```python
from build123d import *

# Parameters (mm, degrees)
SKETCH1_R           = 13.4
BOSS_EXTRUDE1_DEPTH = 56
SKETCH2_W           = 100
SKETCH2_H           = 60
BOSS_EXTRUDE2_DEPTH = 4
SKETCH3_R           = 13.4
CUT_EXTRUDE1_DEPTH  = 25.2
SKETCH4_W           = 25.2
SKETCH4_H           = 25.2
CUT_EXTRUDE2_DEPTH  = 51.2
FILLET1_R           = 5
FILLET2_R           = 5
FILLET4_R           = 3
FILLET5_R           = 3


with BuildPart() as part:
    # Sketch1 → Boss-Extrude1 (new body)
    with BuildSketch(Plane(origin=(0, 0, 0), x_dir=(1, 0, 0), z_dir=(0, 1, 0))):
        Polygon((-65.2, -11.320132013), (-65.2, 44.679867987), (0, 44.679867987), (0, 48.679867987), (-100, 48.679867987), (-100, -11.320132013), align=None)
        with Locations(Location((-82.6, 31.279867987, 0), (0, 0, 270))):
            Circle(SKETCH1_R, mode=Mode.SUBTRACT)
    boss_extrude1 = extrude(amount=BOSS_EXTRUDE1_DEPTH)

    # Sketch2 → Boss-Extrude2 (add)
    with BuildSketch(Plane(origin=(0, 0, 0), x_dir=(1, 0, 0), z_dir=(0, 1, 0))):
        with Locations((-50, 18.679867987)):
            Rectangle(SKETCH2_W, SKETCH2_H)
    boss_extrude2 = extrude(amount=-BOSS_EXTRUDE2_DEPTH)

    # Sketch3 → Cut-Extrude1 (cut)
    with BuildSketch(Plane.XY.offset(11.320132013)):
        with Locations((-82.6, 13.4)):
            Circle(SKETCH3_R)
    cut_extrude1 = extrude(amount=-CUT_EXTRUDE1_DEPTH, mode=Mode.SUBTRACT)

    # Sketch4 → Cut-Extrude2 (cut)
    with BuildSketch(Plane.ZY.offset(100)):
        with Locations((-1.279867987, 43.4)):
            Rectangle(SKETCH4_W, SKETCH4_H)
    cut_extrude2 = extrude(amount=-CUT_EXTRUDE2_DEPTH, mode=Mode.SUBTRACT)

    # Mirror2: Boss-Extrude1, Boss-Extrude2, Cut-Extrude1, Cut-Extrude2 across plane
    add(boss_extrude1.mirror(Plane.ZY))
    add(boss_extrude2.mirror(Plane.ZY))
    add(cut_extrude1.mirror(Plane.ZY), mode=Mode.SUBTRACT)
    add(cut_extrude2.mirror(Plane.ZY), mode=Mode.SUBTRACT)

    # Fillet1
    fillet1_edges = [part.edges().sort_by_distance(p)[0] for p in [
        (0, 0, -44.679867987),
        (-65.2, 0, -16.679867987),
        (-65.2, 28, -44.679867987),
        (65.2, 0, -16.679867987),
        (65.2, 28, -44.679867987),
    ]]
    fillet(fillet1_edges, radius=FILLET1_R)

    # Fillet2
    fillet2_edges = [part.edges().sort_by_distance(p)[0] for p in [
        (-100, 26, -48.679867987),
        (-100, -4, -18.679867987),
        (0, -4, -48.679867987),
        (100, 26, -48.679867987),
        (100, -4, -18.679867987),
    ]]
    fillet(fillet2_edges, radius=FILLET2_R)

    # Fillet4
    fillet4_edges = [part.edges().sort_by_distance(p)[0] for p in [
        (-65.2, 30.8, -1.279867987),
        (-65.2, 43.4, -13.879867987),
        (-82.6, 30.8, -13.879867987),
        (-100, 43.4, -13.879867987),
        (-100, 30.8, -1.279867987),
    ]]
    fillet(fillet4_edges, radius=FILLET4_R)

    # Fillet5
    fillet5_edges = [part.edges().sort_by_distance(p)[0] for p in [
        (100, 43.4, -13.879867987),
        (82.6, 30.8, -13.879867987),
        (100, 30.8, -1.279867987),
        (65.2, 43.4, -13.879867987),
        (65.2, 30.8, -1.279867987),
    ]]
    fillet(fillet5_edges, radius=FILLET5_R)


solid = part.part
```
The model under review builds one solid part; all positions refer to its coordinate system, in mm. A direction names the side the tool comes from. Round coordinates to 2 decimals unless told otherwise and drop trailing zeros. Loops run counter-clockwise (first coordinate to the right, second up) from the corner with the lowest first, then second, coordinate; pieces in that order, holes last. Notation, with made-up numbers: (35.5, 79.5) -> (63.5, 79.5) arc R25 cw to (63.5, 118.5) -> close; hole circle Ø5 at (27.25, 88.5). An arc over 180 degrees is marked (long way). Answer as a JSON object with one key per item and string values. Group by question number.
1) We need section C-C on x = -40. Write out the cut boundary in (y, z).
2) For line 1 (X direction, y = 13, z = -8); line 2 (Z direction, x = 82, y = 42); line 3 (X direction, y = 14, z = -26), list the stretches that pass through material, from the lowest coordinate up. Write a range as [from, to].
3) For pin 1 Ø21.5 at (x, y) = (-82.5, 16) entering from +Z; pin 2 Ø5 at (x, z) = (-75.5, -23.5) entering from +Y; pin 3 Ø8 at (y, z) = (29, -13) entering from -X; pin 4 Ø15.5 at (x, y) = (-29.5, 29) entering from +Z, all flat-tipped, find the tip position at first contact; note any pin that passes through.
4) We need section B-B on z = -8.5. Write out the cut boundary in (x, y), then the cut area to 3 significant figures.
5) For faces 4 (the face through (83, 30.8, 0)), 5 (the face through (1, 0, -15)), 6 (the face through (83, 0, -31)), list the 3-axis set-ups (+Z, -Z, +X, -X, +Y, -Y) from which the entire face can be reached by the end or side of a thin tool; tool diameter is ignored.
6) We need section A-A on y = 49. Write out the cut boundary in (x, z).
7) Mouldability with a two-part tool opening along Z and no side actions: class faces 1 (the face through (1, 29, -48.68)), 2 (the face through (-73.544, 27.608, -41.156)), 3 (the face through (-69.819, 17.425, -1.103)) as released by +Z, released by -Z, zero draft, split by the parting line, or undercut.
8) We need section D-D on z = -26. Write out the cut boundary in (x, y), then the cut area to 3 significant figures.
Result set:
{
 "1": {"outline": "(-4, -43.68) arc R5 ccw to (1, -48.68) -> (56, -48.68) -> (56, -44.68) -> (5, -44.68) arc R5 cw to (0, -39.68) -> (0, 11.32) -> (-4, 11.32) -> close"},
 "2": {"line 1": "[-100, -95.99], [-69.21, -65.2], [65.2, 69.21], [95.99, 100]", "line 2": "[-48.68, -44.67], [-17.89, -13.88]", "line 3": "[-100, -94.92], [-70.28, -65.2], [65.2, 70.28], [94.92, 100]"},
 "3": {"pin 1": "z = -13.88", "pin 2": "y = 0", "pin 3": "x = -100", "pin 4": "z = -44.68"},
 "4": {"outline": "(-100, 1) arc R5 ccw to (-95, -4) -> (95, -4) arc R5 ccw to (100, 1) -> (100, 27.8) arc R3 ccw to (97, 30.8) -> (68.2, 30.8) arc R3 ccw to (65.2, 27.8) -> (65.2, 5) arc R5 cw to (60.2, 0) -> (-60.2, 0) arc R5 cw to (-65.2, 5) -> (-65.2, 27.8) arc R3 ccw to (-68.2, 30.8) -> (-97, 30.8) arc R3 ccw to (-100, 27.8) -> close; hole circle Ø26.8 at (-82.6, 13.4); hole circle Ø26.8 at (82.6, 13.4)", "area": "1,810 mm²"},
 "5": {"face 4": "+Z, +X, -X, +Y", "face 5": "+Z, +Y", "face 6": "+Y"},
 "6": {"outline": "(-100, -43.68) arc R5 ccw to (-95, -48.68) -> (95, -48.68) arc R5 ccw to (100, -43.68) -> (100, -16.88) arc R3 ccw to (97, -13.88) -> (68.2, -13.88) arc R3 ccw to (65.2, -16.88) -> (65.2, -39.68) arc R5 cw to (60.2, -44.68) -> (-60.2, -44.68) arc R5 cw to (-65.2, -39.68) -> (-65.2, -16.88) arc R3 ccw to (-68.2, -13.88) -> (-97, -13.88) arc R3 ccw to (-100, -16.88) -> close; hole circle Ø26.8 at (-82.6, -31.28); hole circle Ø26.8 at (82.6, -31.28)"},
 "7": {"face 1": "released by -Z", "face 2": "undercut", "face 3": "zero draft"},
 "8": {"outline": "(-100, 1) arc R5 ccw to (-95, -4) -> (95, -4) arc R5 ccw to (100, 1) -> (100, 56) -> (94.92, 56) -> (94.92, 0) -> (70.28, 0) -> (70.28, 56) -> (65.2, 56) -> (65.2, 5) arc R5 cw to (60.2, 0) -> (-60.2, 0) arc R5 cw to (-65.2, 5) -> (-65.2, 56) -> (-70.28, 56) -> (-70.28, 0) -> (-94.92, 0) -> (-94.92, 56) -> (-100, 56) -> close", "area": "1,940 mm²"}
}
